Source: CAD feature listing. Evaluate the final solid. Frame: model axes, mm. Face numbers are marked on the shaded views. A direction names the side the tool comes from. Round coordinates to 2 decimals unless told otherwise and drop trailing zeros. Order: outer loops, then holes, each group sorted by start corner. A loop starts at its lowest first (then second) coordinate and runs counter-clockwise, first axis right, second up. Notation, with made-up numbers: (0, 68) - (8, 68) arc R11 cw to (8, 77) - close; hole circle Ø1 at (-4, -39.5). An arc over 180 degrees is marked (long way). Use one line per item in the form item = value. Start each with the question number.
Q1. Cut plane D-D, the plane x = -12. Return the cut outline in (y, z), and give its area (3 significant figures).
Q2. Cut plane B-B, the plane y = 45.5. Return the cut outline in (x, z).
Q3. Cut plane C-C, the plane z = 0. Return the cut outline in (x, y), and give its area (3 significant figures).
Q4. Pin query (flat end, axial travel): pin 1 Ø12 at (x, z) = (27, -4) entering from +Y; pin 2 Ø13.5 at (x, z) = (-42.5, -2) entering from +Y; pin 3 Ø10 at (y, z) = (100, 0) entering from +X. Return the tip coordinate at first contact, or that it passes through.
Q5. Draft query along X for the marked faces 3, 4 and 5. Return one class per face: released by +X, released by -X, zero draft, split by the parting line, or undercut.
Q6. Set-up query: the marked faces 1 and 2. Return all of +Z, -Z, +X, -X, +Y, -Y with unobstructed straight access to the full face (end or side cutting, diameter ignored); none if empty.
Q7. Cut plane A-A, the plane y = 100. Return the cut outline in (x, z).
Q8. Ray query, line 1 (X direction, y = 29, z = -12); line 2 (Y direction, x = -53, z = 0); line 3 (Z direction, x = -18.5, y = 26). Return the intervals inside material, ascending. Write a range as [from, to].
Autodesk Fusion 360 part; units mm, degrees
sketch "Sketch1" plane through (0, 0, 0) normal (0, 1, 0) x (1, 0, 0)
  line L0 (60, 20) -> (-60, 20)
  line L1 (-60, 20) -> (-60, -20)
  line L2 (-60, -20) -> (60, -20)
  line L3 (60, -20) -> (60, 20)
  line L4 (60, 20) -> (-60, -20) construction
  line L5 (-60, 20) -> (60, -20) construction
  line L6 (57, 17) -> (-57, 17)
  line L7 (-57, 17) -> (-57, -17)
  line L8 (-57, -17) -> (57, -17)
  line L9 (57, -17) -> (57, 17)
  line L10 (57, 17) -> (-57, -17) construction
  line L11 (-57, 17) -> (57, -17) construction
  line L12 (-24.159, 17) -> (-21.159, 17)
  line L13 (-21.159, 17) -> (-21.159, -17)
  line L14 (-21.159, -17) -> (-24.159, -17)
  line L15 (-24.159, -17) -> (-24.159, 17)
  line L16 (8.0431, 17) -> (8.0431, -17)
  line L17 (5.0431, -17) -> (5.0431, 17)
  line L18 (8.0431, -17) -> (5.0431, -17)
  line L19 (5.0431, 17) -> (8.0431, 17)
  line L20 (30.4518, 17) -> (33.4518, 17)
  line L21 (33.4518, 17) -> (33.4518, -17)
  line L22 (30.4518, -17) -> (30.4518, 17)
  line L23 (33.4518, -17) -> (30.4518, -17)
  dimension "d1" = 120
  dimension "d2" = 40
  dimension "d3" = 114
  dimension "d4" = 34
  dimension "d20" = 3
  dimension "d21" = 34
  dimension "d26" = 3
  dimension "d27" = 34
  dimension "d28" = 3
  dimension "d29" = 34
extrude "Extrude1" add sketch "Sketch1" along normal blind 80 contours L0 L1 L2 L3 | L6 L8 L20 L21 L22 L23 | L6 L8 L16 L17 L18 L19 | L6 L8 L12 L13 L14 L15 makes body 1
extrude "Extrude2" add sketch "Sketch1" along normal blind 4 contours L6 L8 L9 L21 | L6 L8 L20 L21 L22 L23 | L6 L8 L16 L22 | L6 L8 L16 L17 L18 L19 | L6 L8 L13 L17 | L6 L8 L12 L13 L14 L15 | L6 L7 L8 L15 bodies 1
sketch "Sketch2" plane through (0, 0, 0) normal (1, 0, 0) x (0, 0, -1)
  line L0 (-20, 0) -> (20, 0)
  line L1 (20, 0) -> (20, 80)
  line L2 (20, 80) -> (-20, 80)
  line L3 (-20, 80) -> (-20, 0)
  line L4 (20, 120) -> (-20, 120)
  line L5 (-20, 120) -> (-20, 80)
  line L6 (-20, 80) -> (20, 80)
  line L7 (20, 80) -> (20, 120)
  line L8 (20, 120) -> (-20, 80) construction
  line L9 (-20, 120) -> (20, 80) construction
  line L10 (20, 0) -> (-20, 0)
  line L11 (-20, 0) -> (-20, -40)
  line L12 (-20, -40) -> (20, -40)
  line L13 (20, -40) -> (20, 0)
  line L14 (20, 0) -> (-20, -40) construction
  line L15 (-20, 0) -> (20, -40) construction
  circle A0 centre (0, 100) radius 4.25
  circle A1 centre (0, -20) radius 4.25
  point P0 (0, 100)
  point P1 (0, -20)
  dimension "d9" = 40
  dimension "d10" = 40
  dimension "d11" = 40
  dimension "d12" = 40
  dimension "d13" = 8.5
  dimension "d14" = 8.5
extrude "Extrude3" add sketch "Sketch2" along normal blind -60 and the other way blind 51 contours L0 L1 L2 L3 L6 L10 | L2 L4 L5 L6 L7 bodies 1
fillet "Fillet1" radius 4 2 edges at (60, 40, -20) (60, 40, 20) on bodies 1
copy_body "Body->Comp1" bodies 1 removing the originals makes body 2 in component "item40ToolHoplder-01"
component "item40ToolHoplder-01" placed x (1, 0, 0) y (0, 1, 0) z (0, 0, 1) at (0, 0, 0)
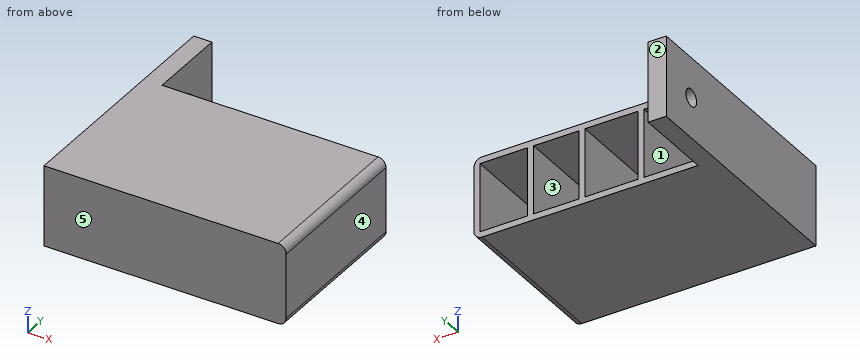
Completed:
q1.outline = (0, -20) - (80, -20) - (80, -17) - (4, -17) - (4, 17) - (80, 17) - (80, 20) - (0, 20) - close
q1.area = 616 mm2
q2.outline = (-60, -20) - (56, -20) arc R4 ccw to (60, -16) - (60, 16) arc R4 ccw to (56, 20) - (-60, 20) - close; hole (-51, -17) - (-24.16, -17) - (-24.16, 17) - (-51, 17) - close; hole (-21.16, -17) - (5.04, -17) - (5.04, 17) - (-21.16, 17) - close; hole (8.04, -17) - (30.45, -17) - (30.45, 17) - (8.04, 17) - close; hole (33.45, -17) - (57, -17) - (57, 17) - (33.45, 17) - close
q3.outline = (-60, 0) - (60, 0) - (60, 80) - (57, 80) - (57, 4) - (33.45, 4) - (33.45, 80) - (30.45, 80) - (30.45, 4) - (8.04, 4) - (8.04, 80) - (5.04, 80) - (5.04, 4) - (-21.16, 4) - (-21.16, 80) - (-24.16, 80) - (-24.16, 4) - (-51, 4) - (-51, 95.75) - (-60, 95.75) - close; (-60, 104.25) - (-51, 104.25) - (-51, 120) - (-60, 120) - close
q3.area = 2,360 mm2
q4.pin_1 = 80
q4.pin_2 = 4
q4.pin_3 = -51
q5.face_3 = undercut
q5.face_4 = released by +X
q5.face_5 = zero draft
q6.face_1 = +Y
q6.face_2 = +Z, -Z, +X, -X, +Y
q7.outline = (-60, -20) - (-51, -20) - (-51, -4.25) - (-60, -4.25) - close; (-60, 4.25) - (-51, 4.25) - (-51, 20) - (-60, 20) - close
q8.line_1 = [-60, -51], [-24.16, -21.16], [5.04, 8.04], [30.45, 33.45], [57, 60]
q8.line_2 = [0, 95.75], [104.25, 120]
q8.line_3 = [-20, -17], [17, 20]
